For this review, take the finished solid that the model builds, in its own axes (mm). A direction names the side the tool comes from. Coordinates: 2 decimals unless noted, no trailing zeros. Write each loop counter-clockwise with the first axis right and the second up, starting at its lowest first coordinate (ties: lowest second). Pieces come first, ordered by that corner, then holes. Notation, with made-up numbers: M 8.5,52 L 53.5,52 A16 ccw 53.5,72 Z; hole C 56.5,75 d2. An arc over 180 degrees is marked long. One line per question, with ' | ' between items.
from build123d import *

# Parameters (mm, degrees)
EXTRUDE_1_DEPTH = 15
SKETCH_2_R      = 12.5
EXTRUDE_2_DEPTH = 15
SKETCH_3_R      = 20
EXTRUDE_3_DEPTH = 12
SKETCH_4_W      = 46
SKETCH_4_H      = 150
EXTRUDE_4_DEPTH = 390
EXTRUDE_5_DEPTH = 15
SKETCH_7_W      = 60
SKETCH_7_H      = 60
EXTRUDE_6_DEPTH = 53
EXTRUDE_7_REACH = 434
SKETCH_8_W      = 90
SKETCH_8_H      = 15
SKETCH_9_R      = 6.75806605
EXTRUDE_8_DEPTH = 22


with BuildPart() as part:
    # ｽｹｯﾁ1 → ﾎﾞｽ - 押し出し1 (new body)
    with BuildSketch(Plane.XY):
        Polygon((0, 0), (90, 0), (90, 300), (25, 300), (25, 85), (0, 85), align=None)
    extrude(amount=EXTRUDE_1_DEPTH)

    # ｽｹｯﾁ2 → ﾎﾞｽ - 押し出し2 (add)
    with BuildSketch(Plane.XY.offset(15)):
        with Locations((57.5, 237.462606559)):
            Circle(SKETCH_2_R)
    extrude(amount=EXTRUDE_2_DEPTH)

    # ｽｹｯﾁ3 → ﾎﾞｽ - 押し出し3 (add)
    with BuildSketch(Plane.XY.offset(30)):
        with Locations((57.5, 237.462606559)):
            Circle(SKETCH_3_R)
    extrude(amount=EXTRUDE_3_DEPTH)

    # ｽｹｯﾁ4 → ﾎﾞｽ - 押し出し4 (add)
    with BuildSketch(Plane(origin=(0, 0, 0), x_dir=(-1, 0, 0), z_dir=(0, 0, -1))):
        with Locations((-57.5, 215)):
            Rectangle(SKETCH_4_W, SKETCH_4_H)
    extrude(amount=EXTRUDE_4_DEPTH)

    # ｽｹｯﾁ6 → ﾎﾞｽ - 押し出し5 (add)
    with BuildSketch(Plane(origin=(0, 0, -390), x_dir=(-1, 0, 0), z_dir=(0, 0, -1))):
        Polygon((-90, 300), (-25, 300), (-25, 85), (0, 85), (0, 0), (-90, 0), align=None)
    extrude(amount=EXTRUDE_5_DEPTH)

    # ｽｹｯﾁ7 → ﾎﾞｽ - 押し出し6 (add)
    with BuildSketch(Plane(origin=(0, 0, -405), x_dir=(-1, 0, 0), z_dir=(0, 0, -1))):
        with Locations((-57.5, 225)):
            Rectangle(SKETCH_7_W, SKETCH_7_H)
    extrude(amount=EXTRUDE_6_DEPTH)

    # ｽｹｯﾁ8 → ﾎﾞｽ - 押し出し7 (add, up to next)
    with BuildSketch(Plane.XY.offset(-390), mode=Mode.PRIVATE) as extrude_7_sk1:
        with Locations((45, 7.5)):
            Rectangle(SKETCH_8_W, SKETCH_8_H)
    extrude_7_tool1 = extrude(extrude_7_sk1.sketch, amount=EXTRUDE_7_REACH, mode=Mode.PRIVATE) - part.part
    add(extrude_7_tool1.solids().sort_by_distance((45, 7.5, -390))[0])

    # ｽｹｯﾁ9 → ﾎﾞｽ - 押し出し8 (add)
    with BuildSketch(Plane.XY.offset(42)):
        with Locations((48.443492705, 245.308936779)):
            Circle(SKETCH_9_R)
    extrude(amount=EXTRUDE_8_DEPTH)


solid = part.part
1) Machinability: for faces 5 (the flat face through (13, 85, -397)), 6 (the flat face through (80.5, 214, -192)), 7 (the flat face through (58, 195, -431)), 8 (the flat face through (58, 255, -431)), 9 (the flat face through (54, 96, 0)), which of the approach directions +Z, -Z, +X, -X, +Y, -Y give a long, thin tool a straight path to every point of the face, cutting with its end or side? Answer none if there is none.
Responses:
face 5: +Z, -Z, -X, +Y | face 6: +X, +Y | face 7: -Z, +X, -X, -Y | face 8: -Z, +X, -X, +Y | face 9: none
2) Insertion check: pin 1 Ø1.5 at (x, y) = (69.5, 116.5) entering from +Z; pin 2 Ø7.5 at (x, z) = (6.5, -400) entering from +Y; pin 3 Ø6 at (x, z) = (28, -296) entering from +Y. Each pin has a flat end and moves straight along its axis. Give the tip position at first contact, or say it passes through.
Responses:
pin 1: z = 15 | pin 2: y = 85 | pin 3: y = 15
3) To check wall thickness, follow line 1 along Z through (x, y) = (50, 88.5); line 2 along Z through (x, y) = (31.5, 242.5); line 3 along Y through (x, z) = (75, -91). State the ranges of each line that lie inside material, in increasing order. Write a range as [from, to].
Responses:
line 1: [-405, -390], [0, 15] | line 2: [-458, -390], [0, 15] | line 3: [0, 15], [140, 290]
4) We need section A-A on z = -240.5. State the section outline as (x, y) points.
Responses:
outline: M 0,0 L 90,0 L 90,15 L 0,15 Z; M 34.5,140 L 80.5,140 L 80.5,290 L 34.5,290 Z
5) We need section C-C on y = 58. State the section outline as (x, z) points, then the cut area to 3 significant figures.
Responses:
outline: M 0,-405 L 90,-405 L 90,-390 L 0,-390 Z; M 0,0 L 90,0 L 90,15 L 0,15 Z | area: 2,700 mm^2
6) The part is to be moulded in two halves that separate along Y. For faces 1 (the cylindrical face through (52.077, 251.007, 52.846)), 2 (the flat face through (0, 14, -243)), 3 (the flat face through (54, 96, -390)), 4 (the flat face through (44, 0, -198)), say which applies: +Y half, -Y half, draft (parallel to the pull), parting line (faces both ways), or undercut.
Responses:
face 1: parting line | face 2: draft | face 3: undercut | face 4: -Y half
7) We need section B-B on y = 145.5. State the section outline as (x, z) points.
Responses:
outline: M 25,-405 L 90,-405 L 90,-390 L 80.5,-390 L 80.5,0 L 90,0 L 90,15 L 25,15 L 25,0 L 34.5,0 L 34.5,-390 L 25,-390 Z
